For this review, take the finished solid that the model builds, in its own axes (mm). A direction names the side the tool comes from. Round coordinates to 2 decimals unless told otherwise and drop trailing zeros. Write each loop counter-clockwise with the first axis right and the second up, starting at its lowest first coordinate (ties: lowest second). Pieces come first, ordered by that corner, then holes. Notation, with made-up numbers: M -3.5,-10 L 0.5,-10 A28 cw 0.5,15 Z; hole C -25,58 d10. An arc over 180 degrees is marked long. Use one line per item in the form item = value. Start each with the question number.
Item 1: For faces 1 (the cylindrical face through (-44.56, -93.005, 0.022)), 2 (the flat face through (-140.712, -29.902, 0.022)), 3 (the flat face through (-117.67, -40.64, -0.02)), list the 3-axis set-ups (+Z, -Z, +X, -X, +Y, -Y) from which the entire face can be reached by the end or side of a thin tool; tool diameter is ignored.
Item 2: Add section A-A (x = -18.5). State the section outline as (y, z) points.
Item 3: Draft analysis for pull direction Y (two halves, no side actions). For faces 4 (the flat face through (-115.801, -43.463, -0.022)), 5 (the flat face through (-112.56, -58.06, 0.02)), 6 (the flat face through (-100.564, -37.731, 0.022)), 7 (the flat face through (-124, 12, -1.588)), state which applies: released by +Y, released by -Y, zero draft, split by the parting line, or undercut.
Item 4: For P1, Ø1, axis at x = -1.5, z = -0.5, coming from the +Y side; P2, Ø1, axis at x = -2.5, z = 0, coming from the -Y side; P3, Ø1, axis at y = -61, z = -0.5, coming from the +X side, all flat-tipped, find the tip position at first contact; note any pin that passes through.
Item 5: Add section B-B (y = 107.5). State the section outline as (x, z) points.
Item 6: Add section C-C (x = -62). State the section outline as (y, z) points, and give its area (3 significant figures).
Item 7: Add section D-D (y = 66). State the section outline as (x, z) points, and give its area (3 significant figures).
Item 8: For line 1 (Y direction, x = -111.5, z = 0.45); line 2 (Y direction, x = -71, z = -1.35); line 3 (Y direction, x = -29, z = 0.75), list the stretches that pass through material, from the lowest coordinate up. Write a range as [from, to].
from build123d import *

# Parameters (mm, degrees)
BOSS_EXTRUDE1_DEPTH = 1.5875
CUT_EXTRUDE1_DEPTH  = 3.175
FILLET1_R           = 8.89
SKETCH4_W           = 218.524279389
SKETCH4_H           = 440.65456999
CUT_EXTRUDE3_DEPTH  = 139.43
BOSS_EXTRUDE2_DEPTH = 1.5875
FILLET2_R           = 12.7
FILLET3_R           = 6.35
SKETCH6_W           = 3.302
SKETCH6_H           = 12.7
CUT_EXTRUDE4_DEPTH  = 4.1750001


with BuildPart() as part:
    # Sketch1 → Boss-Extrude1 (new body, symmetric)
    with BuildSketch(Plane.XY):
        with BuildLine():
            Line((-127.293308919, -32.555250036), (-100.352540556, -59.496018399))
            Line((-100.352540556, -59.496018399), (-100.352540556, -73.509198709))
            ThreePointArc((-100.352540556, -73.509198709), (-79.006783461, -91.825666433), (-54.399250036, -105.449308919))
            ThreePointArc((-54.399250036, -105.449308919), (97.88479172, 119.72879172), (-127.293308919, -32.555250036))
        make_face()
    extrude(amount=BOSS_EXTRUDE1_DEPTH, both=True)

    # Sketch2 → Cut-Extrude1 (cut)
    with BuildSketch(Plane.XY.offset(1.5875)):
        with BuildLine():
            Line((-114.372852664, -23.923091601), (-85.112540556, -53.183403709))
            Line((-85.112540556, -53.183403709), (-85.112540556, -67.215707726))
            ThreePointArc((-85.112540556, -67.215707726), (102.064529488, 90.826663911), (-114.372852664, -23.923091601))
        make_face()
    extrude(amount=-CUT_EXTRUDE1_DEPTH, mode=Mode.SUBTRACT)

    # Fillet1
    fillet1_edges = [part.edges().sort_by_distance(p)[0] for p in [
        (-114.372852664, -23.923091601, 0),
        (-85.112540556, -67.215707726, 0),
        (-85.112540556, -53.183403709, 0),
        (-100.352540556, -73.509198709, -0.79375),
        (-100.352540556, -59.496018399, -0.79375),
        (-127.293308919, -32.555250036, -0.79375),
    ]]
    fillet(fillet1_edges, radius=FILLET1_R)

    # Sketch4 → Cut-Extrude3 (cut, through all)
    with BuildSketch(Plane(origin=(0, 0, 0), x_dir=(0, 0, -1), z_dir=(1, 0, 0))):
        with Locations((12.98164036, 12.468370851)):
            Rectangle(SKETCH4_W, SKETCH4_H)
    extrude(amount=CUT_EXTRUDE3_DEPTH, mode=Mode.SUBTRACT)

    # Sketch5 → Boss-Extrude2 (add, symmetric)
    with BuildSketch(Plane.XY):
        with BuildLine():
            Line((-100.344096462, -70.2778643), (-93.131982579, -63.067144592))
            Line((-93.131982579, -63.067144592), (-135.386236526, -2.54))
            ThreePointArc((-135.386236526, -2.54), (-145.549369809, -8.667691803), (-155.542666772, -15.068621483))
            Line((-155.542666772, -15.068621483), (-100.344096462, -70.2778643))
        make_face()
    extrude(amount=BOSS_EXTRUDE2_DEPTH, both=True)

    # Fillet2
    fillet2_edges = [part.edges().sort_by_distance(p)[0] for p in [
        (-136.181300165, -3.005917211, 0),
    ]]
    fillet(fillet2_edges, radius=FILLET2_R)

    # Fillet3
    fillet3_edges = [part.edges().sort_by_distance(p)[0] for p in [
        (-100.344096462, -70.2778643, -0.79375),
    ]]
    fillet(fillet3_edges, radius=FILLET3_R)

    # Sketch6 → Cut-Extrude4 (cut, through all)
    with BuildSketch(Plane(origin=(0, 0, -1.5875), x_dir=(-1, 0, 0), z_dir=(0, 0, -1))):
        with Locations((1.651, 157.734)):
            Rectangle(SKETCH6_W, SKETCH6_H)
        Polygon((109.598496198, 91.009030044), (111.278220029, 88.078029687), (122.297018363, 94.392780931), (120.617294532, 97.323781288), align=None)
        Polygon((108.408719805, -39.179754441), (110.102498062, -36.256853407), (126.58502269, -45.808234558), (124.891244433, -48.731135592), align=None)
        with Locations((1.651, -114.046)):
            Rectangle(SKETCH6_W, SKETCH6_H)
    extrude(amount=-CUT_EXTRUDE4_DEPTH, mode=Mode.SUBTRACT)


solid = part.part
Calculated:
q1.face_1 = +Z, -Z, +X
q1.face_2 = +Z, -Z, -X, -Y
q1.face_3 = +Z, -Z
q2.outline = M -115.34,-1.59 L -99.95,-1.59 L -99.95,1.59 L -115.34,1.59 Z; M 143.64,-1.59 L 159.03,-1.59 L 159.03,1.59 L 143.64,1.59 Z
q3.face_4 = undercut
q3.face_5 = released by -Y
q3.face_6 = undercut
q3.face_7 = zero draft
q4.P1 = 151.38
q4.P2 = -107.7
q4.P3 = -85.11
q5.outline = M -108.75,-1.59 L -88.54,-1.59 L -88.54,1.59 L -108.75,1.59 Z
q6.outline = M -101.93,-1.59 L -84.61,-1.59 L -84.61,1.59 L -101.93,1.59 Z; M 128.29,-1.59 L 145.61,-1.59 L 145.61,1.59 L 128.29,1.59 Z
q6.area = 110 mm^2
q7.outline = M -131.2,-1.59 L -115,-1.59 L -115,1.59 L -131.2,1.59 Z
q7.area = 51.4 mm^2
q8.line_1 = [-59.12, -40.97], [-37.07, -26.8], [74.22, 88.21], [92.1, 103.88]
q8.line_2 = [-96.99, -78.83], [122.52, 140.68]
q8.line_3 = [-113.51, -97.88], [141.57, 157.2]
